```python
from build123d import *

# Parameters (mm, degrees)
ESBO_O1_W                  = 63.3
ESBO_O1_H                  = 52
ESBO_O1_R                  = 11.5
ESBO_O1_R_2                = 1.75
ESBO_O1_R_3                = 1.65
RESSALTO_EXTRUS_O1_DEPTH   = 25
ESBO_O2_W                  = 13.3
ESBO_O2_H                  = 21
CORTE_EXTRUS_O1_DEPTH      = 27
CORTE_EXTRUS_O1_DEPTH_BACK = 27
RESSALTO_EXTRUS_O2_DEPTH   = 4
ESBO_O4_W                  = 24
ESBO_O4_H                  = 16
ESBO_O4_R                  = 1.65
RESSALTO_EXTRUS_O3_DEPTH   = 4
ESBO_O5_R                  = 5.25
CORTE_EXTRUS_O2_DEPTH      = 1
ESBO_O6_R                  = 5.25
CORTE_EXTRUS_O3_DEPTH      = 1


with BuildPart() as part:
    # Esboço1 → Ressalto-extrusão1 (new body)
    with BuildSketch(Plane.XY):
        with Locations((-9.65, 0)):
            Rectangle(ESBO_O1_W, ESBO_O1_H)
        Circle(ESBO_O1_R, mode=Mode.SUBTRACT)
        with Locations((-15.5, 15.5)):
            Circle(ESBO_O1_R_2, mode=Mode.SUBTRACT)
        with Locations((15.5, 15.5)):
            Circle(ESBO_O1_R_2, mode=Mode.SUBTRACT)
        with Locations((15.5, -15.5)):
            Circle(ESBO_O1_R_2, mode=Mode.SUBTRACT)
        with Locations((-15.5, -15.5)):
            Circle(ESBO_O1_R_2, mode=Mode.SUBTRACT)
        with Locations((-31.3, -15.5)):
            Circle(ESBO_O1_R_3, mode=Mode.SUBTRACT)
        with Locations((-31.3, 15.5)):
            Circle(ESBO_O1_R_3, mode=Mode.SUBTRACT)
    extrude(amount=RESSALTO_EXTRUS_O1_DEPTH)

    # Esboço2 → Corte-extrusão1 (cut, two sides)
    with BuildSketch(Plane(origin=(0, 0, 0), x_dir=(1, 0, 0), z_dir=(0, 1, 0))) as corte_extrus_o1_sk:
        with Locations((-34.65, -14.5)):
            Rectangle(ESBO_O2_W, ESBO_O2_H)
        Polygon((-23, -25), (22, -25), (22, -4), align=None)
        Polygon((-23, -25), (22, -4), (-23, -4), (-28, -4), (-28, -25), align=None)
    extrude(amount=CORTE_EXTRUS_O1_DEPTH, mode=Mode.SUBTRACT)
    extrude(corte_extrus_o1_sk.sketch, amount=-CORTE_EXTRUS_O1_DEPTH_BACK, mode=Mode.SUBTRACT)

    # Esboço3 → Ressalto-extrusão2 (add)
    with BuildSketch(Plane(origin=(0, 26, 0), x_dir=(1, 0, 0), z_dir=(0, 1, 0))):
        Polygon((22, -4), (-17.3, -24), (-21.3, -24), (-21.3, -4), align=None)
    ressalto_extrus_o2 = extrude(amount=-RESSALTO_EXTRUS_O2_DEPTH)

    # Esboço4 → Ressalto-extrusão3 (add)
    with BuildSketch(Plane.ZY.offset(21.3)):
        with Locations((12, 30)):
            Rectangle(ESBO_O4_W, ESBO_O4_H)
        with Locations((14, 32)):
            Circle(ESBO_O4_R, mode=Mode.SUBTRACT)
    ressalto_extrus_o3 = extrude(amount=-RESSALTO_EXTRUS_O3_DEPTH)

    # Espelhar1: Ressalto-extrusão2, Ressalto-extrusão3 across plane
    add(ressalto_extrus_o2.mirror(Plane.ZX))
    add(ressalto_extrus_o3.mirror(Plane.ZX))

    # Esboço5 → Corte-extrusão2 (cut)
    with BuildSketch(Plane.ZY.offset(21.3)):
        with Locations((14, -32)):
            Circle(ESBO_O5_R)
        with Locations((14, 32)):
            Circle(ESBO_O5_R)
    extrude(amount=-CORTE_EXTRUS_O2_DEPTH, mode=Mode.SUBTRACT)

    # Esboço6 → Corte-extrusão3 (cut)
    with BuildSketch(Plane.XY.offset(4)):
        with Locations((-31.3, 15.5)):
            Circle(ESBO_O6_R)
        with Locations((-31.3, -15.5)):
            Circle(ESBO_O6_R)
    extrude(amount=-CORTE_EXTRUS_O3_DEPTH, mode=Mode.SUBTRACT)


solid = part.part
```
Verification items for the finished model (mm, model axes). A direction names the side the tool comes from. Round coordinates to 2 decimals unless told otherwise and drop trailing zeros. Order: outer loops, then holes, each group sorted by start corner. A loop starts at its lowest first (then second) coordinate and runs counter-clockwise, first axis right, second up. Notation, with made-up numbers: (1, -30) - (35, -30) arc R12 cw to (35, -16) - close; hole circle Ø2 at (-3.75, 77). An arc over 180 degrees is marked (long way). Use CSV: the item, a comma, the result in double quotes. Start each with the question number.
1) Section check C-C, the plane x = -9.5. Record the cut outline in (y, z).
2) Access from +Z, -Z, +X, -X, +Y, -Y to the whole of each face (thin tool, end or side, straight path). Record for faces 4 (the flat face through (-31, 26, 2)), 5 (the flat face through (-17.3, 32, 12)), 6 (the cylindrical face through (-26.3, 17.1, 3.5)), 7 (the cylindrical face through (-20.807, -31.769, 8.755)), 8 (the flat face through (-19, -30, 24)).
3) Section check D-D, the plane y = -15.5. Record the cut outline in (x, z), plus the area to 3 significant figures.
4) Section check B-B, the plane z = 14. Record the cut outline in (x, y).
5) Section check A-A, the plane y = 0. Record the cut outline in (x, z), plus the area to 3 significant figures.
6) Go/stop test with flat-tipped pins: P1, Ø4, axis at x = 9.5, z = 7, coming from the +Y side; P2, Ø3, axis at x = -31, y = 16.5, coming from the +Z side; P3, Ø7, axis at x = 10, z = 14, coming from the -Y side. Record where each tip stops, or that it passes through.
7) Thickness scan on L1, parallel to Y at x = -21, z = 14; L2, parallel to X at y = -15.5, z = 2.3; L3, parallel to Y at x = 3.5, z = 10.5. Record the ranges inside material, lowest first.
8) Mould release check, pull along Z, two halves, no side actions. Record for faces 1 (the flat face through (-4, 22, 12)), 2 (the flat face through (2.625, -24.028, 13.86)), 3 (the flat face through (-20.3, -34, 14)): +Z half, -Z half, draft (parallel to the pull), parting line (faces both ways), or undercut.
Answers:
1,outline,"(-26, 0) - (-6.48, 0) - (-6.48, 4) - (-22, 4) - (-22, 20.03) - (-26, 20.03) - close; (6.48, 0) - (26, 0) - (26, 20.03) - (22, 20.03) - (22, 4) - (6.48, 4) - close"
2,face 4,"+Z, -Z, -X, +Y"
2,face 5,"+Z, -Z, +X, +Y"
2,face 6,"+Z"
2,face 7,"-X"
2,face 8,"+Z, +X, -X, +Y, -Y"
3,outline,"(-41.3, 0) - (-32.95, 0) - (-32.95, 3) - (-36.55, 3) - (-36.55, 4) - (-41.3, 4) - close; (-29.65, 0) - (-17.25, 0) - (-17.25, 4) - (-26.05, 4) - (-26.05, 3) - (-29.65, 3) - close; (-13.75, 0) - (13.75, 0) - (13.75, 4) - (-13.75, 4) - close; (17.25, 0) - (22, 0) - (22, 4) - (17.25, 4) - close"
3,area,"205 mm²"
4,outline,"(-21.3, -38) - (-17.3, -38) - (-17.3, -33.65) - (-20.3, -33.65) - (-20.3, -37.25) - (-21.3, -37.25) - close; (-21.3, -26.75) - (-20.3, -26.75) - (-20.3, -30.35) - (-17.3, -30.35) - (-17.3, -26) - (2.35, -26) - (2.35, -22) - (-21.3, -22) - close; (-21.3, 22) - (2.35, 22) - (2.35, 26) - (-17.3, 26) - (-17.3, 30.35) - (-20.3, 30.35) - (-20.3, 26.75) - (-21.3, 26.75) - close; (-21.3, 37.25) - (-20.3, 37.25) - (-20.3, 33.65) - (-17.3, 33.65) - (-17.3, 38) - (-21.3, 38) - close"
5,outline,"(-41.3, 0) - (-11.5, 0) - (-11.5, 4) - (-41.3, 4) - close; (11.5, 0) - (22, 0) - (22, 4) - (11.5, 4) - close"
5,area,"161 mm²"
6,P1,"stops at y = 26"
6,P2,"stops at z = 3"
6,P3,"stops at y = -26"
7,L1,"y = -38 to -37.25, -26.75 to -22, 22 to 26.75, 37.25 to 38"
7,L2,"x = -41.3 to -32.95, -29.65 to -17.25, -13.75 to 13.75, 17.25 to 22"
7,L3,"y = -26 to -22, 22 to 26"
8,face 1,"draft"
8,face 2,"+Z half"
8,face 3,"undercut"
